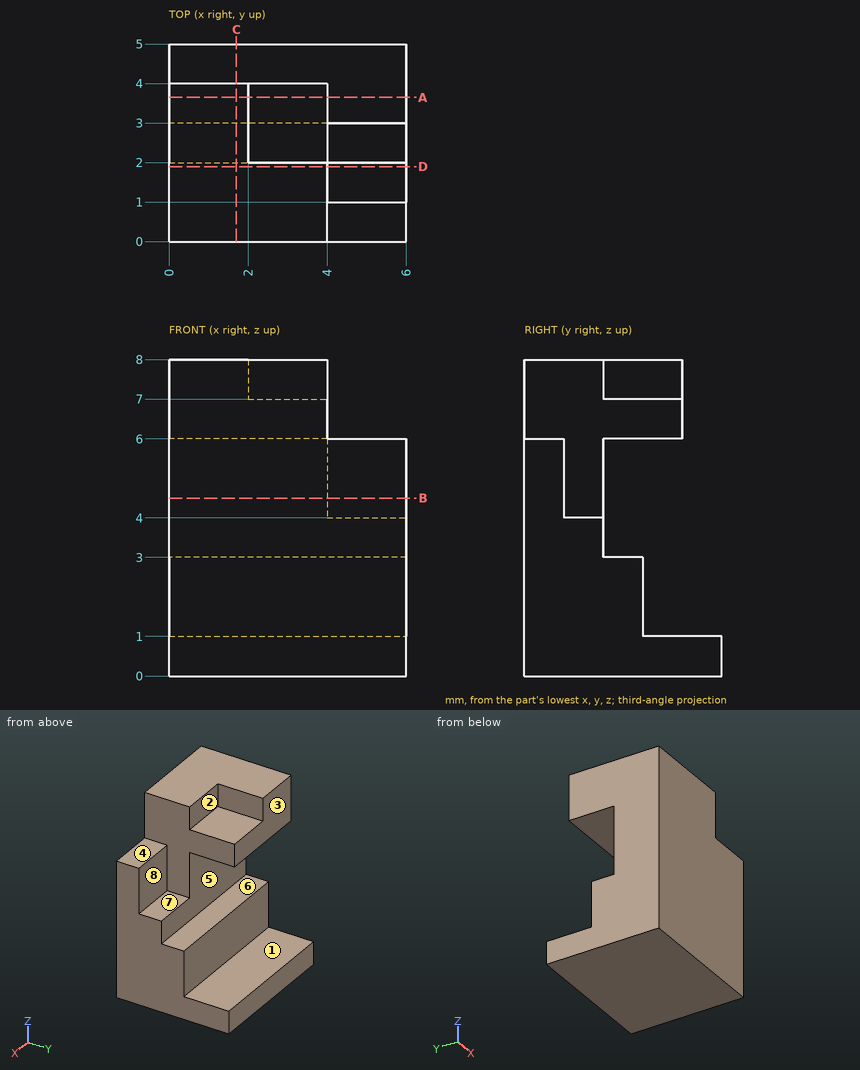
Geometry: see drawing. Coordinates: mm, zero at the bounding-box minimum. A direction names the side the tool comes from. Round coordinates to 2 decimals unless told otherwise and drop trailing zeros. Loops run counter-clockwise (first coordinate to the right, second up) from the corner with the lowest first, then second, coordinate; pieces in that order, holes last.
(1) Section query B-B (z = 4.5). Output: boundary loops of the cut face in (x, y).
From the geometry:
outline: (0, 0) - (6, 0) - (6, 1) - (4, 1) - (4, 2) - (0, 2) - close
(2) Section query A-A (y = 3.65). Output: boundary loops of the cut face in (x, z).
From the geometry:
outline: (0, 0) - (6, 0) - (6, 1) - (0, 1) - close; (0, 6) - (4, 6) - (4, 7) - (2, 7) - (2, 8) - (0, 8) - close
(3) Contact query for flat-ended pins moving along their axis: pin 1 Ø0.9 at (x, z) = (2.5, 4.5) entering from +Y; pin 2 Ø2 at (x, z) = (5, 6.5) entering from -Y; pin 3 Ø3 at (x, z) = (3.5, 4) entering from +Y; pin 4 Ø0.6 at (x, z) = (4.5, 5) entering from +Y. Output: stop coordinate, or through.
From the geometry:
pin 1: stops at y = 2
pin 2: stops at y = 0
pin 3: stops at y = 3
pin 4: stops at y = 1
(4) Access query for the marked faces 1, 2, 3 and 4. Directions: +Z, -Z, +X, -X, +Y, -Y. A direction counts if a zero-diameter tool reaches every point of the face in a straight line with its end or side. Return the directions, or none.
From the geometry:
face 1: +X, -X, +Y
face 2: +Z, +X, +Y
face 3: +Z, +X, -X, +Y
face 4: +Z, +X, +Y, -Y
(5) Section query D-D (y = 1.9). Output: boundary loops of the cut face in (x, z), and give its area (3 significant figures).
From the geometry:
outline: (0, 0) - (6, 0) - (6, 4) - (4, 4) - (4, 8) - (0, 8) - close
area: 40.0 mm2
(6) Material intervals for probe 1 along Y at (x, z) = (4.7, 5.5); probe 2 along X at (y, z) = (1.55, 4.5); probe 3 along Y at (x, z) = (0.35, 5.5), sorted ascending.
From the geometry:
probe 1: y = 0 to 1
probe 2: x = 0 to 4
probe 3: y = 0 to 2
(7) Pull-direction query (Z, two-part tool) for the marked faces 5, 6, 7 and 8; classes: +Z half, -Z half, draft (parallel to the pull), parting line (faces both ways), or undercut.
From the geometry:
face 5: undercut
face 6: undercut
face 7: +Z half
face 8: draft
(8) Section query C-C (x = 1.7). Output: boundary loops of the cut face in (y, z), and give its area (3 significant figures).
From the geometry:
outline: (0, 0) - (5, 0) - (5, 1) - (3, 1) - (3, 3) - (2, 3) - (2, 6) - (4, 6) - (4, 8) - (0, 8) - close
area: 25.0 mm2
